Design review of the part built by this model. Coordinates are the model's own, in mm. Coordinates: 2 decimals unless noted, no trailing zeros. Loops run counter-clockwise (first coordinate to the right, second up) from the corner with the lowest first, then second, coordinate; pieces in that order, holes last. Notation, with made-up numbers: (31.5, -32) - (89.5, -32) arc R26 ccw to (89.5, -8) - close; hole circle Ø9 at (48, 45.25). An arc over 180 degrees is marked (long way). Use one line per item in the form item = value. Start each with the question number.
(1) The part is to be moulded in two halves that separate along Y. For faces 1 (the face through (-40.524, -12.933, 9.126)), 2 (the face through (-1, -16, 9)), 3 (the face through (-1, 0, 0)), say which applies: pulls with the +Y half, pulls with the -Y half, needs draft (parallel to the pull), parting line crosses it, or undercut.
(2) For L1, parallel to Y at x = -39, z = 7 (3 decimals); L2, parallel to Y at x = 38, z = 5; L3, parallel to X at y = -12, z = 1, list the stretches that pass through material, from the lowest coordinate up.
(3) Add section B-B (y = -13). State the section outline as (x, z) points (3 decimals).
(4) Add section A-A (x = 39). State the section outline as (y, z) points (3 decimals).
```python
from build123d import *

# Parameters (mm, degrees)
SKETCH_1_W               = 85
SKETCH_1_H               = 32
EXTRUDE_1_DEPTH          = 18
SKETCH_2_R               = 1.525
CUT_EXTRUDE_1_DEPTH      = 1
CUT_EXTRUDE_1_DEPTH_BACK = 19


with BuildPart() as part:
    # 草图1 → 凸台-拉伸1 (new body)
    with BuildSketch(Plane.XY):
        Rectangle(SKETCH_1_W, SKETCH_1_H)
    extrude(amount=EXTRUDE_1_DEPTH)

    # 草图2 → 切除-拉伸1 (cut, two sides)
    with BuildSketch(Plane.XY.offset(18)) as cut_extrude_1_sk:
        with Locations((39, 13)):
            Circle(SKETCH_2_R)
        with Locations((39, -13)):
            Circle(SKETCH_2_R)
        with Locations((-39, -13)):
            Circle(SKETCH_2_R)
        with Locations((-39, 13)):
            Circle(SKETCH_2_R)
    extrude(amount=CUT_EXTRUDE_1_DEPTH, mode=Mode.SUBTRACT)
    extrude(cut_extrude_1_sk.sketch, amount=-CUT_EXTRUDE_1_DEPTH_BACK, mode=Mode.SUBTRACT)


solid = part.part
```
Computed values:
q1.face_1 = undercut
q1.face_2 = pulls with the -Y half
q1.face_3 = needs draft
q2.L1 = -16 to -14.525, -11.475 to 11.475, 14.525 to 16
q2.L2 = -16 to -14.15, -11.85 to 11.85, 14.15 to 16
q2.L3 = -42.5 to -40.15, -37.85 to 37.85, 40.15 to 42.5
q3.outline = (-42.5, 0) - (-40.525, 0) - (-40.525, 18) - (-42.5, 18) - close; (-37.475, 0) - (37.475, 0) - (37.475, 18) - (-37.475, 18) - close; (40.525, 0) - (42.5, 0) - (42.5, 18) - (40.525, 18) - close
q4.outline = (-16, 0) - (-14.525, 0) - (-14.525, 18) - (-16, 18) - close; (-11.475, 0) - (11.475, 0) - (11.475, 18) - (-11.475, 18) - close; (14.525, 0) - (16, 0) - (16, 18) - (14.525, 18) - close
